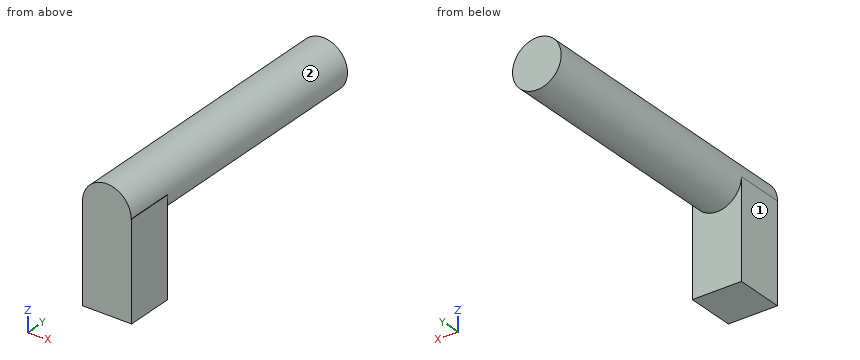
from build123d import *

# Parameters (mm, degrees)
F1_R     = 12.7
F2_DEPTH = 152.4
F4_DEPTH = 25.4


with BuildPart() as f2:
    # F1 (on face) → F2 (new body)
    with BuildSketch(Plane.XZ):
        with Locations((-27.7367867529, 61.1216872931)):
            Circle(F1_R)
    extrude(amount=F2_DEPTH)

    # F3 (on face) → F4 (join)
    with BuildSketch(Plane.XZ.offset(152.4)):
        with BuildLine():
            Line((-14.8034961894, 61.1216872931), (-15.0367867529, 61.1216872931))
            ThreePointArc((-15.0367867529, 61.1216872931), (-27.7367867529, 48.4216872931), (-40.4367867529, 61.1216872931))
            Line((-40.4367867529, 61.1216872931), (-40.4367867529, 10.3216872931))
            Line((-40.4367867529, 10.3216872931), (-14.8034961894, 10.3216872931))
            Line((-14.8034961894, 10.3216872931), (-14.8034961894, 61.1216872931))
        make_face()
    extrude(amount=-F4_DEPTH)


solid = f2.part
The model under review builds one solid part; all positions refer to its coordinate system, in mm. Face numbers are marked on the shaded views. A direction names the side the tool comes from. Round coordinates to 2 decimals unless told otherwise and drop trailing zeros. Order: outer loops, then holes, each group sorted by start corner. A loop starts at its lowest first (then second) coordinate and runs counter-clockwise, first axis right, second up. Notation, with made-up numbers: (77.5, -32.75) -> (107.5, -32.75) arc R25 cw to (107.5, -1.75) -> close; hole circle Ø4 at (55.25, 19.25). An arc over 180 degrees is marked (long way). Return JSON: item names as keys, results as strings.
1. Take a section at D-D (y = -109.5). Write out the cut boundary in (x, z).
Answer block:
{"outline": "circle Ø25.4 at (-27.74, 61.12)"}
2. For the marked faces 1 and 2, list the 3-axis set-ups (+Z, -Z, +X, -X, +Y, -Y) from which the entire face can be reached by the end or side of a thin tool; tool diameter is ignored.
Answer block:
{"face 1": "+Z, -Z, -X, +Y, -Y", "face 2": "+Y"}
3. Take a section at B-B (z = 44). Write out the cut boundary in (x, y), then the cut area to 3 significant figures.
Answer block:
{"outline": "(-40.44, -152.4) -> (-14.8, -152.4) -> (-14.8, -127) -> (-40.44, -127) -> close", "area": "651 mm²"}
4. For L1, parallel to Y at x = -36.25, z = 27.5; L2, parallel to Z at x = -17.75, y = -34.5; L3, parallel to Z at x = -21.5, y = -90.5, list the stretches that pass through material, from the lowest coordinate up. Write a range as [from, to].
Answer block:
{"L1": "y = [-152.4, -127]", "L2": "z = [53.28, 68.97]", "L3": "z = [50.06, 72.18]"}
5. Insertion check: P1, Ø1, axis at x = -18.5, z = 24.5, coming from the +Y side; P2, Ø4, axis at y = -111, z = 44.5, coming from the +X side; P3, Ø1.5, axis at x = -29.5, y = -21, coming from the +Z side; P4, Ø12, axis at y = -84.5, z = 46.5, coming from the +X side. Each pin has a flat end and moves straight along its axis. Give the tip position at first contact, or say it passes through.
Answer block:
{"P1": "stops at y = -127", "P2": "passes through", "P3": "stops at z = 73.78", "P4": "stops at x = -18.41"}
6. Take a section at C-C (x = -37). Write out the cut boundary in (y, z), then the cut area to 3 significant figures.
Answer block:
{"outline": "(-152.4, 10.32) -> (-127, 10.32) -> (-127, 52.43) -> (0, 52.43) -> (0, 69.81) -> (-152.4, 69.81) -> close", "area": "3,720 mm²"}
7. Take a section at A-A (y = -133). Write out the cut boundary in (x, z).
Answer block:
{"outline": "(-40.44, 10.32) -> (-14.8, 10.32) -> (-14.8, 61.12) -> (-15.04, 61.12) arc R12.7 ccw to (-40.44, 61.12) -> close"}
